Autodesk Inventor part; units mm, degrees
ref_plane "YZ Plane" through (0, 0, 0) normal (1, 0, 0) x (0, 1, 0)
ref_plane "XZ Plane" through (0, 0, 0) normal (0, 1, 0) x (-1, 0, 0)
ref_plane "XY Plane" through (0, 0, 0) normal (0, 0, 1) x (1, 0, 0)
sketch "Sketch1" plane through (0, 0, 0) normal (0, 0, 1) x (1, 0, 0)
  circle A0 centre (0, 0) radius 20
  dimension "d0" = 40
extrude "Extrusion1" add sketch "Sketch1" along normal mid plane 8
sketch "Sketch2" plane through (0, 0, -4) normal (0, 0, -1) x (-1, 0, 0)
  line L0 (-20, 0) -> (20, 0) construction
  line L1 (-20, -5) -> (20, -5)
  line L2 (20, 5) -> (-20, 5)
  arc A0 (-20, 5) -> (-20, -5) centre (-20, 0) ccw
  arc A1 (20, -5) -> (20, 5) centre (20, 0) ccw
  line L3 (0, 0) -> (40, 0) construction
  dimension "d3" = 20
  dimension "d4" = 0
  dimension "d5" = 10
extrude "Extrusion2" cut sketch "Sketch2" against normal blind 4
sketch "Sketch6" plane through (0, 0, 4) normal (0, 0, 1) x (1, 0, 0)
  line L0 (-28, 0) -> (28, 0)
  arc A0 (14.5, 1.5) -> (10.0623, 3) centre (9.9997, -4.4997) ccw
  line L1 (14.5, 1.5) -> (14.5, 0)
  arc A1 (10.0623, -3) -> (14.5, -1.5) centre (9.9997, 4.4997) ccw
  line L2 (14.5, -1.5) -> (14.5, 0)
  arc A2 (7.8679, 12.2718) -> (3.9283, 9.7375) centre (9.7527, 5.0125) ccw
  line L3 (7.8679, 12.2718) -> (9.0406, 11.3366)
  line L4 (10.2133, 10.4013) -> (9.0406, 11.3366)
  arc A3 (8.6192, 5.9966) -> (10.2133, 10.4013) centre (2.7166, 10.6236) ccw
  arc A4 (-4.6889, 13.8027) -> (-5.1639, 9.1425) centre (2.1618, 10.7502) ccw
  line L5 (-4.6889, 13.8027) -> (-3.2266, 14.1365)
  line L6 (-1.7642, 14.4702) -> (-3.2266, 14.1365)
  arc A5 (0.6857, 10.4776) -> (-1.7642, 14.4702) centre (-6.6121, 8.7477) ccw
  arc A6 (-13.7149, 4.9399) -> (-10.3675, 1.663) centre (-7.057, 8.3928) ccw
  line L7 (-13.7149, 4.9399) -> (-13.064, 6.2913)
  line L8 (-12.4132, 7.6428) -> (-13.064, 6.2913)
  arc A7 (-7.7642, 7.0688) -> (-12.4132, 7.6428) centre (-10.9617, 0.2846) ccw
  arc A8 (-12.4132, -7.6428) -> (-7.7642, -7.0688) centre (-10.9617, -0.2846) ccw
  line L9 (-12.4132, -7.6428) -> (-13.064, -6.2913)
  line L10 (-13.7149, -4.9399) -> (-13.064, -6.2913)
  arc A9 (-10.3675, -1.663) -> (-13.7149, -4.9399) centre (-7.057, -8.3928) ccw
  arc A10 (-1.7642, -14.4702) -> (0.6857, -10.4776) centre (-6.6121, -8.7477) ccw
  line L11 (-1.7642, -14.4702) -> (-3.2266, -14.1365)
  line L12 (-4.6889, -13.8027) -> (-3.2266, -14.1365)
  arc A11 (-5.1639, -9.1425) -> (-4.6889, -13.8027) centre (2.1618, -10.7502) ccw
  arc A12 (10.2133, -10.4013) -> (8.6192, -5.9966) centre (2.7166, -10.6236) ccw
  line L13 (10.2133, -10.4013) -> (9.0406, -11.3366)
  line L14 (7.8679, -12.2718) -> (9.0406, -11.3366)
  arc A13 (3.9283, -9.7375) -> (7.8679, -12.2718) centre (9.7527, -5.0125) ccw
  arc A14 (10.0623, 3) -> (8.6192, 5.9966) centre (0, 0) ccw
  arc A15 (3.9283, 9.7375) -> (0.6857, 10.4776) centre (0, 0) ccw
  arc A16 (-5.1639, 9.1425) -> (-7.7642, 7.0688) centre (0, 0) ccw
  arc A17 (-10.3675, 1.663) -> (-10.3675, -1.663) centre (0, 0) ccw
  arc A18 (-7.7642, -7.0688) -> (-5.1639, -9.1425) centre (0, 0) ccw
  arc A19 (0.6857, -10.4776) -> (3.9283, -9.7375) centre (0, 0) ccw
  arc A20 (8.6192, -5.9966) -> (10.0623, -3) centre (0, 0) ccw
  dimension "d33" = 1.5
  dimension "d34" = 3
  dimension "d35" = 7.5
  dimension "d36" = 14.5
  dimension "d39" = 360
extrude "Extrusion4" add sketch "Sketch6" along normal blind 4
properties part number "3d-tandwiel"
Here's how the part is built. I have some questions about the finished solid (model axes, mm). A direction names the side the tool comes from. Give positions to 0.01 mm unless a question says otherwise; leave off trailing zeros. Order: outer loops, then holes, each group sorted by start corner. A loop starts at its lowest first (then second) coordinate and runs counter-clockwise, first axis right, second up. Notation, with made-up numbers: M 25.5,33 L 34.5,33 A19 cw 34.5,52 Z; hole C 83.25,3.25 d6. An arc over 180 degrees is marked long. Answer as a JSON object with one key per item and string values. Group by question number.
1) On a 3-axis mill with a long thin cutter (end or side, diameter ignored), from which of +Z, -Z, +X, -X, +Y, -Y can I reach the whole of each face in a straight line? I mean faces 4 (the flat face through (0, 5, -2)), 5 (the cylindrical face through (2.314, 10.242, 5.972)), 6 (the flat face through (-9, -9, 4)), 7 (the cylindrical face through (9.47, -4.535, 5.972)), 8 (the cylindrical face through (-10.5, 0, 6)). Say none if no direction works.
2) I'm going to push flat-ended pins straight in: pin 1 Ø5 at (y, z) = (-6.5, 2.5) entering from +X; pin 2 Ø3.5 at (y, z) = (-0.5, 7) entering from +X; pin 3 Ø3 at (x, z) = (-3.5, -1.5) entering from +Y. Where does each tip first touch, or does it pass through?
3) Suppose I cut it at B-B, the plane y = 0. Write out the boundary of the cut face in (x, z).
4) We'd pull the mould along Y, two halves only. Please class faces 1 (the cylindrical face through (5.667, 11.302, 5.972)), 2 (the cylindrical face through (19.076, -6.007, -0.056)), 3 (the cylindrical face through (-12.28, 3.01, 5.97)): pulls with the +Y half, pulls with the -Y half, needs draft (parallel to the pull), parting line crosses it, or undercut.
5) Suppose I cut it at D-D, the plane x = 7. Write out the boundary of the cut face in (y, z) (3 decimals).
6) Please list where these lines run through material, in increasing order: L1, parallel to Z at x = -2, y = 4.5; L2, parallel to Z at x = 5.5, y = -12; L3, parallel to Y at x = 16.5, z = -0.5. Write a range as [from, to].
7) Suppose I cut it at C-C, the plane x = 0. Write out the boundary of the cut face in (y, z).
Results found:
{
 "1": {"face 4": "-Z, +X, -X", "face 5": "+Z, +Y", "face 6": "+Z", "face 7": "+Z, +X", "face 8": "+Z, -X"},
 "2": {"pin 1": "x = 19.6", "pin 2": "x = 14.5", "pin 3": "y = 19.9"},
 "3": {"outline": "M -20,0 L 20,0 L 20,4 L 14.5,4 L 14.5,8 L -10.5,8 L -10.5,4 L -20,4 Z"},
 "4": {"face 1": "pulls with the +Y half", "face 2": "parting line crosses it", "face 3": "undercut"},
 "5": {"outline": "M -18.735,-4 L -5,-4 L -5,0 L 5,0 L 5,-4 L 18.735,-4 L 18.735,4 L 11.989,4 L 11.989,8 L -11.989,8 L -11.989,4 L -18.735,4 Z"},
 "6": {"L1": "[0, 8]", "L2": "[-4, 4]", "L3": "[-11.3, -5], [5, 11.3]"},
 "7": {"outline": "M -20,-4 L -5,-4 L -5,0 L 5,0 L 5,-4 L 20,-4 L 20,4 L 12.29,4 L 12.29,8 L -12.29,8 L -12.29,4 L -20,4 Z"}
}
